Design review of the part shown in the three views and the two pictorial views. Dimensions are in mm from the part's minimum x, y and z. Give positions to 0.01 mm unless a question says otherwise; leave off trailing zeros. Loops run counter-clockwise (first coordinate to the right, second up) from the corner with the lowest first, then second, coordinate; pieces in that order, holes last. Notation, with made-up numbers: (36.25, -30.5) - (93.25, -30.5) arc R18 cw to (93.25, -13.5) - close; hole circle Ø7 at (13.5, -18.5). An arc over 180 degrees is marked (long way). Answer in a Markdown table with one row per item.
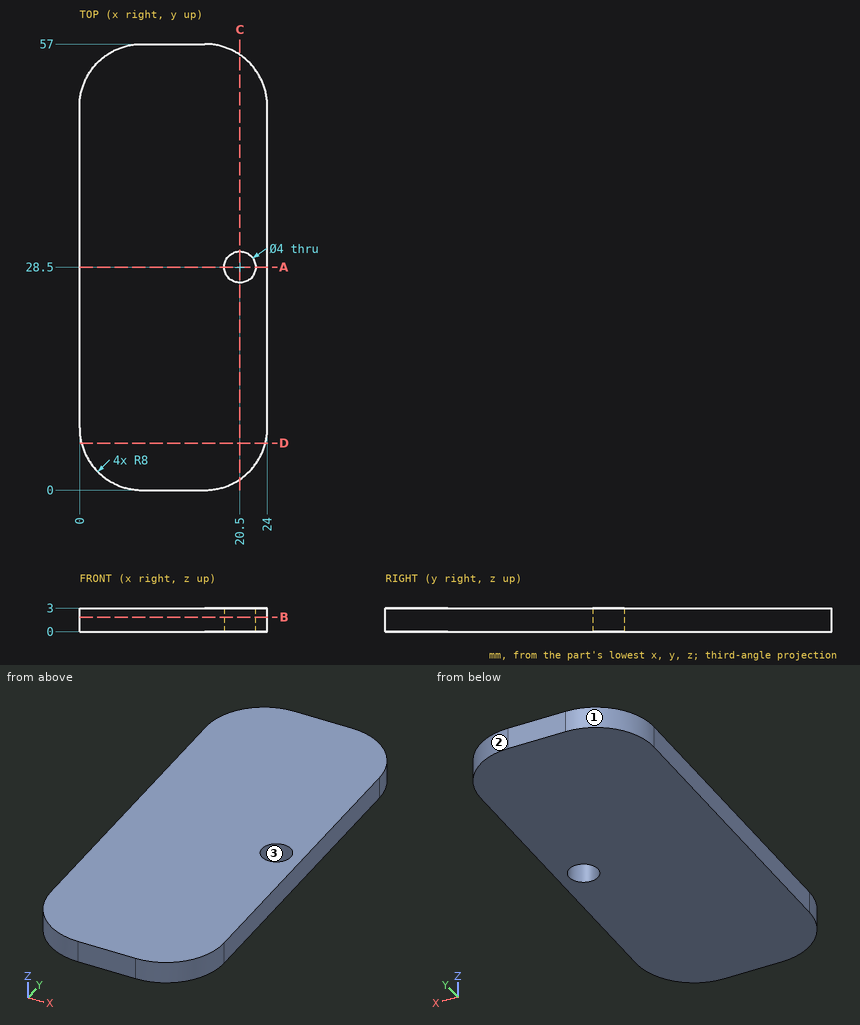
1. Clearance check with flat-ended pins moving along their axes: pin 1 (10 mm diameter, centred on x = 18, y = 24.5, fed in from -Z); pin 2 (3 mm diameter, centred on x = 20.5, y = 28.5, fed in from -Z). State where each tip first meets the part, or that it passes through.
Values:
| item | result |
|---|---|
| pin 1 | stops at z = 0 |
| pin 2 | passes through |
2. Mouldability with a two-part tool opening along X and no side actions: class the marked faces 1, 2 and 3 as released by +X, released by -X, zero draft, split by the parting line, or undercut.
Values:
| item | result |
|---|---|
| face 1 | released by -X |
| face 2 | released by +X |
| face 3 | undercut |
3. Wall thickness on line 1 (X direction, y = 28.5, z = 1.95); line 2 (Y direction, x = 20.5, z = 0.95); line 3 (Y direction, x = 19.5, z = 0.8): over which ranges is each line inside the solid? List them lowest first. Write a range as [from, to].
Values:
| item | result |
|---|---|
| line 1 | x = [0, 18.5], [22.5, 24] |
| line 2 | y = [1.39, 26.5], [30.5, 55.61] |
| line 3 | y = [0.81, 26.77], [30.23, 56.19] |
4. We need section D-D, the plane y = 6. Give the boundary of the cut face in (x, z), and give its area (3 significant figures).
Values:
| item | result |
|---|---|
| outline | (0.25, 0) - (23.75, 0) - (23.75, 3) - (0.25, 3) - close |
| area | 70.5 mm^2 |
5. We need section A-A, the plane y = 28.5. Give the boundary of the cut face in (x, z), and give its area (3 significant figures).
Values:
| item | result |
|---|---|
| outline | (0, 0) - (18.5, 0) - (18.5, 3) - (0, 3) - close; (22.5, 0) - (24, 0) - (24, 3) - (22.5, 3) - close |
| area | 60.0 mm^2 |
6. We need section C-C, the plane x = 20.5. Give the boundary of the cut face in (y, z), and give its area (3 significant figures).
Values:
| item | result |
|---|---|
| outline | (1.39, 0) - (26.5, 0) - (26.5, 3) - (1.39, 3) - close; (30.5, 0) - (55.61, 0) - (55.61, 3) - (30.5, 3) - close |
| area | 151 mm^2 |
7. We need section B-B, the plane z = 1.85. Give the boundary of the cut face in (x, y), and give its area (3 significant figures).
Values:
| item | result |
|---|---|
| outline | (0, 8) arc R8 ccw to (8, 0) - (16, 0) arc R8 ccw to (24, 8) - (24, 49) arc R8 ccw to (16, 57) - (8, 57) arc R8 ccw to (0, 49) - close; hole circle Ø4 at (20.5, 28.5) |
| area | 1,300 mm^2 |
